Autodesk Inventor part; units mm, degrees
ref_plane "YZ Plane" through (0, 0, 0) normal (1, 0, 0) x (0, 1, 0)
ref_plane "XZ Plane" through (0, 0, 0) normal (0, 1, 0) x (-1, 0, 0)
ref_plane "XY Plane" through (0, 0, 0) normal (0, 0, 1) x (1, 0, 0)
sketch "Sketch1" plane through (0, 0, 0) normal (0, 1, 0) x (-1, 0, 0)
  line L0 (0, 0) -> (110, 0)
  line L1 (110, 0) -> (110, -180)
  line L2 (0, -180) -> (0, 0)
  line L3 (67.5, -200) -> (42.5, -200)
  line L4 (67.5, -200) -> (110, -180)
  line L5 (42.5, -200) -> (0, -180)
  dimension "d2" = 180
  dimension "d38" = 25
extrude "Extrusion1" add sketch "Sketch1" along normal blind 2
sketch "Sketch2" plane through (0, 2, 0) normal (0, 1, 0) x (1, 0, 0)
  line L0 (0, 180) -> (-110, 180)
  line L1 (-110, 180) -> (-110, 0)
  line L2 (0, 180) -> (-110, 180)
  line L3 (-110, 180) -> (-110, 0)
  line L4 (-110, 0) -> (0, 0)
  line L5 (0, 0) -> (0, 180)
  line L6 (0, 0) -> (0, 180)
  line L7 (-110, 0) -> (0, 0)
  line L8 (-2, 2) -> (-108, 2)
  line L9 (-108, 2) -> (-108, 178)
  line L10 (-108, 178) -> (-2, 178)
  line L11 (-2, 178) -> (-2, 2)
extrude "Extrusion2" add sketch "Sketch2" along normal blind 50
sketch "Sketch3" plane through (-108, 2, -2) normal (1, 0, 0) x (0, 0, -1)
  line L0 (0, 50) -> (176, 50)
  line L1 (65, 40) -> (65, 0)
  line L2 (176, 0) -> (0, 0)
  line L3 (67, 40) -> (67, 0)
  line L4 (67, 0) -> (65, 0)
  line L5 (97, 40) -> (97, 0)
  line L6 (97, 0) -> (99, 0)
  line L7 (99, 0) -> (99, 40)
  line L8 (65, 40) -> (67, 40)
  line L9 (99, 40) -> (97, 40)
  point P0 (-2, -2)
  point P1 (67, 0)
extrude "Extrusion3" add sketch "Sketch3" along normal up to next
sketch "Sketch4" plane through (0, 2, 0) normal (0, 1, 0) x (1, 0, 0)
  line L0 (-108, 69) -> (-2, 69)
  line L1 (-90, 69) -> (-90, 99)
  line L2 (-108, 99) -> (-2, 99)
  line L3 (-2, 69) -> (-2, 99)
  line L4 (-20, 69) -> (-20, 99)
  line L5 (-20, 99) -> (-90, 99)
  line L6 (-90, 69) -> (-20, 69)
  point P0 (0, 0)
extrude "Extrusion4" cut sketch "Sketch4" against normal up to next contours L1 L2 L4 L0
sketch "Sketch5" plane through (-108, 2, -178) normal (1, 0, 0) x (0, 0, -1)
  line L0 (-111, 0) -> (-111, 40)
  line L1 (-111, 0) -> (-176, 0)
  circle A0 centre (-132, 21) radius 11
  circle A1 centre (-147.5, 36.5) radius 1.5
  circle A2 centre (-116.5, 36.5) radius 1.5
  circle A3 centre (-147.5, 36.5) radius 1.5
  circle A4 centre (-147.5, 5.5) radius 1.5
  circle A5 centre (-116.5, 5.5) radius 1.5
  point P0 (-178, -2)
extrude "Extrusion5" cut sketch "Sketch5" along normal through all both and the other way through all
sketch "Sketch6" plane through (-108, 2, -178) normal (0, 0, 1) x (1, 0, 0)
  line L0 (106, 0) -> (106, 50)
  line L1 (106, 50) -> (0, 50)
  line L2 (0, 50) -> (0, 0)
  line L3 (0, 0) -> (106, 0)
  line L4 (106, 0) -> (106, 50)
  point P0 (108, -2)
extrude "Extrusion6" cut sketch "Sketch6" against normal up to next
sketch "Sketch7" plane through (0, 2, 0) normal (0, 1, 0) x (1, 0, 0)
  line L0 (-67.5, 200) -> (-110, 180)
  line L1 (-110, 180) -> (-67.5, 200)
  line L2 (-67.5, 200) -> (-42.5, 200)
  line L3 (0, 180) -> (-42.5, 200)
  line L4 (-42.5, 200) -> (0, 180)
  line L5 (-67.5, 198) -> (-42.5, 198)
  line L6 (-99.9511, 182.7289) -> (-67.5, 198)
  line L7 (-99.9511, 182.7289) -> (-108, 178.9412)
  line L8 (-108, 180) -> (-108, 101)
  line L9 (-108, 180) -> (-110, 180)
  line L10 (-21.25, 188) -> (-42.5, 198)
  line L11 (-21.25, 188) -> (-2, 178.9412)
  line L12 (-2, 101) -> (-2, 180)
  line L13 (-2, 180) -> (0, 180)
  line L14 (0, 180) -> (-42.5, 200)
  line L15 (-42.5, 200) -> (-67.5, 200)
  line L16 (-42.5, 200) -> (-67.5, 200)
  line L17 (-110, 180) -> (-110, 0)
  line L18 (-67.5, 200) -> (-110, 180)
  point P0 (0, 0)
extrude "Extrusion7" add sketch "Sketch7" along normal up to surface (50 mm away)
sketch "Sketch8" plane through (-42.5, 0, -200) normal (0, 0, -1) x (-1, 0, 0)
  line L0 (0, 0) -> (25, 0)
  line L1 (8, 39.5) -> (17, 39.5)
  line L2 (17, 39.5) -> (17, 30.5)
  line L3 (17, 30.5) -> (8, 30.5)
  line L4 (8, 30.5) -> (8, 39.5)
  line L5 (8, 39.5) -> (17, 30.5) construction
  line L6 (17, 39.5) -> (8, 30.5) construction
  point P0 (-42.5, 0)
  dimension "d48" = 9
  dimension "d49" = 9
extrude "Extrusion8" cut sketch "Sketch8" against normal blind 2
sketch "Sketch9" plane through (0, 2, 0) normal (0, 1, 0) x (1, 0, 0)
  line L0 (-108, 2) -> (-108, 178.9412)
  line L1 (-108, 2) -> (-106, 2)
  line L2 (-106, 2) -> (-106, 4)
  line L3 (-106, 4) -> (-108, 4)
  line L4 (-108, 4) -> (-108, 2)
  line L5 (-2, 2) -> (-108, 2)
  line L6 (-2, 2) -> (-4, 2)
  line L7 (-4, 2) -> (-4, 4)
  line L8 (-4, 4) -> (-2, 4)
  line L9 (-2, 4) -> (-2, 2)
  line L10 (-67.5, 198) -> (-108, 178.9412)
  line L11 (-106, 178.9412) -> (-106, 176.9412)
  line L12 (-106, 176.9412) -> (-108, 176.9412)
  line L13 (-108, 176.9412) -> (-108, 178.9412)
  line L14 (-106, 178.9412) -> (-106, 179.8824)
  line L15 (-108, 178.9412) -> (-108, 101)
  line L16 (-108, 178.9412) -> (-106, 179.8824)
  line L17 (-2, 178.9412) -> (-2, 2)
  line L18 (-4, 178.9412) -> (-4, 176.9412)
  line L19 (-4, 176.9412) -> (-2, 176.9412)
  line L20 (-2, 176.9412) -> (-2, 178.9412)
  line L21 (-4, 178.9412) -> (-4, 179.8824)
  line L22 (-2, 178.9412) -> (-42.5, 198)
  line L23 (-4, 179.8824) -> (-2, 178.9412)
  line L24 (-4, 179.8824) -> (-2, 178.9412)
  line L25 (-67.5, 198) -> (-108, 178.9412)
  line L26 (-67.5, 198) -> (-67.5, 196)
  line L27 (-67.5, 196) -> (-71.75, 196)
  line L28 (-42.5, 198) -> (-67.5, 198)
  line L29 (-42.5, 198) -> (-42.5, 196)
  line L30 (-42.5, 196) -> (-38.25, 196)
  line L31 (-42.5, 198) -> (-38.25, 196)
  line L32 (-71.75, 196) -> (-67.5, 198)
  line L33 (-55, 2) -> (-53, 2)
  line L34 (-53, 2) -> (-53, 4)
  line L35 (-53, 4) -> (-57, 4)
  line L36 (-57, 4) -> (-57, 2)
  line L37 (-57, 2) -> (-55, 2)
  point P0 (0, 0)
extrude "Extrusion9" add sketch "Sketch9" along normal blind 48 contours L0 L3 L2 L1 | L36 L35 L34 L5 | L0 L10 L14 L11 L12 | L7 L8 L9 L5 | L10 L26 L27 | L22 L30 L29 | L19 L18 L21 L22 L17
sketch "Sketch10" plane through (-108, 42, -101) normal (0, 1, 0) x (1, 0, 0)
  line L0 (0, 0) -> (106, 0)
  line L1 (0, -2) -> (106, -2)
  line L2 (106, 0) -> (104, 0)
  line L3 (104, 0) -> (104, -2)
  line L4 (104, -2) -> (106, -2)
  line L5 (106, -2) -> (106, 0)
  line L6 (106, -32) -> (106, -34)
  line L7 (106, -32) -> (104, -32)
  line L8 (104, -32) -> (104, -34)
  line L9 (104, -34) -> (106, -34)
  line L10 (106, -34) -> (106, -32)
  line L11 (106, -34) -> (0, -34)
  line L12 (0, -32) -> (18, -32)
  line L13 (0, -34) -> (2, -34)
  line L14 (2, -34) -> (2, -32)
  line L15 (2, -32) -> (0, -32)
  line L16 (0, -32) -> (0, -34)
  line L17 (0, -2) -> (0, 0)
  line L18 (0, 0) -> (2, 0)
  line L19 (2, 0) -> (2, -2)
  line L20 (2, -2) -> (0, -2)
  line L21 (0, -2) -> (0, 0)
  point P0 (108, -101)
  point P1 (2, -34)
  point P2 (2, -2)
  point P3 (2, 0)
extrude "Extrusion10" add sketch "Sketch10" along normal blind 8 contours L0 L19 L1 L17 | L0 L5 L1 L3 | L11 L16 L12 L14 | L6 L9 L8 L7
sketch "Sketch12" plane through (0, 2, 0) normal (0, 1, 0) x (1, 0, 0)
  line L0 (-106, 99) -> (-4, 99)
  line L1 (-55, 99) -> (-100, 99)
  line L2 (-100, 99) -> (-100, 69)
  line L3 (-108, 101) -> (-2, 101)
  line L4 (-100, 99) -> (-70, 99) construction
  line L5 (-108, 99) -> (-108, 69)
  line L6 (-108, 99) -> (-100, 99)
  line L7 (-100, 99) -> (-100, 69)
  line L8 (-100, 69) -> (-108, 69)
  line L9 (-108, 69) -> (-108, 99)
  line L10 (-10, 99) -> (-10, 69)
  line L11 (-2, 99) -> (-2, 69)
  line L12 (-2, 99) -> (-10, 99)
  line L13 (-10, 99) -> (-10, 69)
  line L14 (-10, 69) -> (-2, 69)
  line L15 (-2, 69) -> (-2, 99)
  point P0 (0, 0)
extrude "Extrusion12" add sketch "Sketch12" along normal blind 6
sketch "Sketch13" plane through (0, 2, 0) normal (0, 1, 0) x (1, 0, 0)
  line L0 (-42.5, 198) -> (-67.5, 198)
  circle A0 centre (-61.75, 183) radius 1.5
  circle A1 centre (-48.25, 183) radius 1.5
  point P0 (0, 0)
extrude "Extrusion13" cut sketch "Sketch13" against normal through all
properties part number "Robot"
Read the model definition and answer for the solid it produces. Units are mm, in the model's axes. A direction names the side the tool comes from. Coordinates: 2 decimals unless noted, no trailing zeros. Write each loop counter-clockwise with the first axis right and the second up, starting at its lowest first coordinate (ties: lowest second). Pieces come first, ordered by that corner, then holes. Notation, with made-up numbers: (-14.75, -26) - (21.25, -26) arc R20 cw to (21.25, -5) - close; hole circle Ø7 at (7.25, 2.25). An arc over 180 degrees is marked (long way). One line per question, with ' | ' between items.
Q1. Find section D-D, the plane y = 23. State how many separate pieces and enclosed holes the cut face has, plus the area to 3 significant figures.
Result set:
separate pieces: 2 | enclosed holes: 2 | area: 1,520 mm^2
Q2. Consider L1, parallel to Y at x = -1.5, z = -30.5; L2, parallel to Z at x = -54.5, y = 38.5; L3, parallel to X at y = 14.5, z = -108.5. Determine where each line is inside the solid, lowest interval first. Write a range as [from, to].
Result set:
L1: [0, 6], [9, 37], [40, 52] | L2: [-101, -99], [-69, -67], [-4, 0] | L3: [-110, -108], [-2, 0]
Q3. For faces 1 (the flat face through (-104, 8, -84)), 2 (the flat face through (0, 26, -91)), determine the directions among +Z, -Z, +X, -X, +Y, -Y from which every point of the face is accessible in a straight line to the end or side of a thin tool.
Result set:
face 1: +Y | face 2: +Z, -Z, +X, +Y, -Y
Q4. Find section B-B, the plane z = -46. Write down the section's boundary in (x, y).
Result set:
outline: (-110, 0) - (0, 0) - (0, 12) - (-2, 12) - (-2, 2) - (-108, 2) - (-108, 12) - (-110, 12) - close; (-110, 34) - (-108, 34) - (-108, 52) - (-110, 52) - close; (-2, 34) - (0, 34) - (0, 52) - (-2, 52) - close
Q5. Find section A-A, the plane z = -87.5. Write down the section's boundary in (x, y), plus the area to 3 significant figures.
Result set:
outline: (-110, 0) - (-90, 0) - (-90, 2) - (-100, 2) - (-100, 8) - (-108, 8) - (-108, 52) - (-110, 52) - close; (-20, 0) - (0, 0) - (0, 52) - (-2, 52) - (-2, 8) - (-10, 8) - (-10, 2) - (-20, 2) - close | area: 376 mm^2
Q6. Each of these flat-tipped pins is pushed along its axis until it touches: P1, Ø1.5, axis at x = -82.5, y = 6, coming from the -Z side; P2, Ø0.6, axis at x = -3, z = -99.5, coming from the +Y side; P3, Ø2.5, axis at y = 7.5, z = -61.5, coming from the -X side; P4, Ø0.6, axis at x = -50.5, z = -68, coming from the +Y side. Where does it stop, or does it pass through?
Result set:
P1: z = -193.29 | P2: y = 50 | P3: through | P4: y = 42
Q7. Determine the mould class of faces 3 (the flat face through (-54, 0, -121)), 4 (the flat face through (-70, 26, -196)), 5 (the flat face through (-54, 26, 0)), 6 (the flat face through (-55, 26, -200)) for opening direction Z: +Z half, -Z half, draft (parallel to the pull), parting line (faces both ways), or undercut.
Result set:
face 3: draft | face 4: undercut | face 5: +Z half | face 6: -Z half
Q8. Find section C-C, the plane z = -13. Write down the section's boundary in (x, y), plus the area to 3 significant figures.
Result set:
outline: (-110, 0) - (0, 0) - (0, 52) - (-2, 52) - (-2, 2) - (-108, 2) - (-108, 52) - (-110, 52) - close | area: 420 mm^2
